Source: three-view drawing plus pictorial views. Frame: mm from the lowest corner of the part. A direction names the side the tool comes from. Give positions to 0.01 mm unless a question says otherwise; leave off trailing zeros. Loops run counter-clockwise (first coordinate to the right, second up) from the corner with the lowest first, then second, coordinate; pieces in that order, holes last.
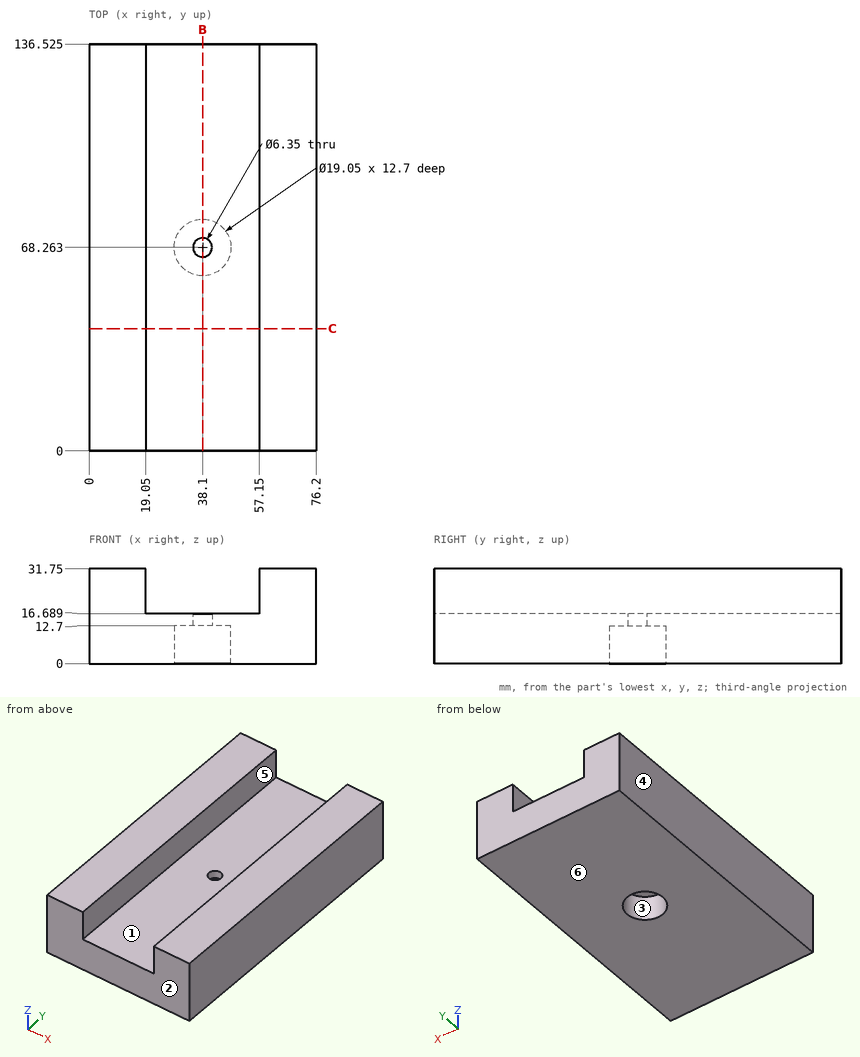
(1) Cut plane B-B (x = 38.1). Return the cut outline in (y, z) (1 decimal).
Values follow:
outline: (0, 0) - (58.7, 0) - (58.7, 12.7) - (65.1, 12.7) - (65.1, 16.7) - (0, 16.7) - close; (71.4, 12.7) - (77.8, 12.7) - (77.8, 0) - (136.5, 0) - (136.5, 16.7) - (71.4, 16.7) - close
(2) Reachability of the marked faces 1 and 2 from +Z, -Z, +X, -X, +Y, -Y: full face, straight path, thin tool, end or side. Return the list, or none.
Values follow:
face 1: +Z, +Y, -Y
face 2: +Z, -Z, +X, -X, -Y
(3) Cut plane C-C (y = 41). Return the cut outline in (x, z), and give its area (3 significant figures).
Values follow:
outline: (0, 0) - (76.2, 0) - (76.2, 31.75) - (57.15, 31.75) - (57.15, 16.69) - (19.05, 16.69) - (19.05, 31.75) - (0, 31.75) - close
area: 1,850 mm2
(4) Pin query (flat end, axial travel): pin 1 Ø12 at (y, z) = (93, 17) entering from -X; pin 2 Ø5.5 at (x, y) = (35.5, 67) entering from -Z; pin 3 Ø19 at (x, y) = (37.5, 72) entering from +Z; pin 4 Ø4 at (x, z) = (31, 20) entering from +Y. Return the tip coordinate at first contact, or that it passes through.
Values follow:
pin 1: stops at x = 0
pin 2: stops at z = 12.7
pin 3: stops at z = 16.69
pin 4: passes through
(5) Ray query, probe 1 along X at (y, z) = (107, 28); probe 2 along Y at (x, z) = (38.1, 8.5) (1 decimal); probe 3 along Y at (x, z) = (38.1, 13.9) (1 decimal). Return the intervals inside material, ascending.
Values follow:
probe 1: x = 0 to 19.05, 57.15 to 76.2
probe 2: y = 0 to 58.7, 77.8 to 136.5
probe 3: y = 0 to 65.1, 71.4 to 136.5
(6) Mould query, pull axis X, two halves, no side actions, for the marked faces 3, 4, 5 and 6. Classes: +X half, -X half, draft (parallel to the pull), parting line (faces both ways), or undercut.
Values follow:
face 3: undercut
face 4: -X half
face 5: undercut
face 6: draft
